```python
from build123d import *

# Parameters (mm, degrees)
BOSS_EXTRUDE1_DEPTH      = 135
BOSS_EXTRUDE1_DEPTH_BACK = 135
BOSS_EXTRUDE2_DEPTH      = 140


with BuildPart() as part:
    # Sketch1 → Boss-Extrude1 (new, two sides: drawn at the far end of the back side and taken through both)
    with BuildSketch(Plane(origin=(0, 0, 0), x_dir=(0, 0, -1), z_dir=(1, 0, 0)).offset(-BOSS_EXTRUDE1_DEPTH_BACK)):
        Polygon((-350, 90), (-350, 0), (350, 0), (350, 280), (230, 280), (230, 90), (140, 90), (60, 260), (-140, 260), (-220, 90), align=None)
    extrude(amount=BOSS_EXTRUDE1_DEPTH + BOSS_EXTRUDE1_DEPTH_BACK)

    # Sketch3 → Boss-Extrude2 (add)
    with BuildSketch(Plane.ZY.offset(135)):
        Polygon((350, 90), (350, 130), (180.554272517, 173.822170901), (220, 90), align=None)
        Polygon((-230, 280), (-230, 90), (-140, 90), (-70.054249548, 238.634719711), align=None)
    extrude(amount=-BOSS_EXTRUDE2_DEPTH)


solid = part.part
```
Geometry check sheet. Reference: the model listing, model coordinates, mm. A direction names the side the tool comes from. Give positions to 0.01 mm unless a question says otherwise; leave off trailing zeros. Order: outer loops, then holes, each group sorted by start corner. A loop starts at its lowest first (then second) coordinate and runs counter-clockwise, first axis right, second up.
1. Section check D-D, the plane x = 115.5. Enter the section's corners in (y, z), and give its area (3 significant figures).
2. Access from +Z, -Z, +X, -X, +Y, -Y to the whole of each face (thin tool, end or side, straight path). Record for faces 1 (the face through (-65.98, 259.03, -148.91)), 2 (the face through (69, 90, -186)), 3 (the face through (28.11, 195.08, 170.55)).
3. Section check A-A, the plane x = -48. Enter the section's corners in (y, z).
4. Release check for a two-part mould opening along Z. For faces 4 (the face through (-135, 111, -5)), 5 (the face through (-2, 138, -350)), 6 (the face through (5, 186, -169)), 7 (the face through (-2, 50, 350)) record: pulls with the +Z half, pulls with the -Z half, needs draft (parallel to the pull), parting line crosses it, or undercut.
5. Gauge pin test, flat ends, axial feed: pin 1 Ø25 at (y, z) = (122, 257) entering from +X; pin 2 Ø2 at (x, z) = (-32.5, -224) entering from -Y. Record the tip position at first contact, or that the pin passes through.
6. Thickness scan on L1, parallel to Z at x = 48, y = 258; L2, parallel to Y at x = 99.5, z = 12.5; L3, parallel to X at y = 227.5, z = -132.5. Record the ranges inside material, lowest first.
7. Section check B-B, the plane y = 115. Enter the section's corners in (x, z).
8. Section check C-C, the plane z = 125.5. Enter the section's corners in (x, y).
Values follow:
1. outline: (0, -350) - (280, -350) - (280, -230) - (90, -230) - (90, -140) - (260, -60) - (260, 140) - (90, 220) - (90, 350) - (0, 350) - close
1. area: 133,000 mm2
2. face 1: +X, -X, +Y
2. face 2: +X, +Y
2. face 3: +Z, +X, +Y
3. outline: (0, -350) - (280, -350) - (280, -230) - (238.63, -70.05) - (260, -60) - (260, 140) - (173.82, 180.55) - (130, 350) - (0, 350) - close
4. face 4: needs draft
4. face 5: pulls with the -Z half
4. face 6: undercut
4. face 7: pulls with the +Z half
5. pin 1: stops at x = 5
5. pin 2: stops at y = 0
6. L1: z = -350 to -230, -60.94 to 140.94
6. L2: y = 0 to 260
6. L3: x = -135 to 5
7. outline: (-135, -350) - (135, -350) - (135, -230) - (5, -230) - (5, -128.24) - (135, -128.24) - (135, 208.24) - (5, 208.24) - (5, 350) - (-135, 350) - close
8. outline: (-135, 0) - (135, 0) - (135, 260) - (-135, 260) - close
